Input: part model. Units: mm. Frame: model coordinates. A direction names the side the tool comes from. Coordinates: 2 decimals unless noted, no trailing zeros. Write each loop counter-clockwise with the first axis right and the second up, starting at its lowest first coordinate (ties: lowest second). Pieces come first, ordered by that corner, then holes. Notation, with made-up numbers: M -30.5,59 L 1.5,59 A27 cw 1.5,92 Z; hole C 74,63 d4. An arc over 180 degrees is marked long. Use one line per item in the form item = value.
from build123d import *

# Parameters (mm, degrees)
F0_W     = 30
F0_H     = 154.5
F0_H_2   = 30
F0_W_2   = 190
F0_H_3   = 184.5
F1_DEPTH = 800
F3_DEPTH = 50
F5_DEPTH = 50


with BuildPart() as f1:
    # F0 (on Front) → F1 (new body)
    with BuildSketch(Plane.XZ):
        with Locations((-15, 77.25)):
            Rectangle(F0_W, F0_H)
        with Locations((-15, 169.5)):
            Rectangle(F0_W, F0_H_2)
        with Locations((-125, 169.5)):
            Rectangle(F0_W_2, F0_H_2)
        with Locations((-235, 169.5)):
            Rectangle(F0_W, F0_H_2)
        with Locations((-235, 261.75)):
            Rectangle(F0_W, F0_H)
        with Locations((-235, 354)):
            Rectangle(F0_W, F0_H_2)
        with Locations((-345, 354)):
            Rectangle(F0_W_2, F0_H_2)
        with Locations((-455, 354)):
            Rectangle(F0_W, F0_H_2)
        with Locations((-455, 446.25)):
            Rectangle(F0_W, F0_H)
        with Locations((-455, 538.5)):
            Rectangle(F0_W, F0_H_2)
        with Locations((-565, 538.5)):
            Rectangle(F0_W_2, F0_H_2)
        with Locations((-675, 538.5)):
            Rectangle(F0_W, F0_H_2)
        with Locations((-675, 645.75)):
            Rectangle(F0_W, F0_H_3)
    extrude(amount=F1_DEPTH)

    # F2 (on face) → F3 (join)
    with BuildSketch(Plane.XZ.offset(800)):
        Polygon((-690, 738), (-690, 523.5), (-590, 439.636364), (-590, 700.658275), (-590, 738), align=None)
        Polygon((-590, 439.636364), (-690, 523.5), (-690, 439.636364), align=None)
        Polygon((-590, 700.658275), (-590, 439.636364), (-100, 28.704545), (-100, 289.726456), align=None)
        Polygon((-100, 289.726456), (-100, 28.704545), (-100, -200), (0, -200), (0, 289.726456), align=None)
    extrude(amount=F3_DEPTH)

    # F4 (on face) → F5 (join)
    with BuildSketch(Plane(origin=(0, 0, 0), x_dir=(-1, 0, 0), z_dir=(0, 1, 0))):
        Polygon((0, 289.726456), (0, -200), (100, -200), (100, 28.704545), (100, 289.726456), align=None)
        Polygon((100, 289.726456), (100, 28.704545), (590, 439.636364), (590, 700.658275), align=None)
        Polygon((590, 700.658275), (590, 439.636364), (690, 439.636364), (690, 738), (590, 738), align=None)
    extrude(amount=F5_DEPTH)


solid = f1.part
(1) Section query B-B on x = -635.5. Return the cut outline in (y, z), plus the area to 3 significant figures.
Computed:
outline = M -850,439.64 L -800,439.64 L -800,523.5 L 0,523.5 L 0,439.64 L 50,439.64 L 50,738 L 0,738 L 0,553.5 L -800,553.5 L -800,738 L -850,738 Z
area = 53,800 mm^2
(2) First-contact query: pin 1 Ø8 at (y, z) = (-607.5, 487) entering from +X; pin 2 Ø8 at (y, z) = (-238.5, 349) entering from -X; pin 3 Ø1.5 at (y, z) = (-654, 598.5) entering from +X. Flat tips, straight axial feed; report the tip coordinate or a pass-through.
Computed:
pin_1 = -440
pin_2 = -470
pin_3 = -660
(3) Section query C-C on y = -97. Return the cut outline in (x, z).
Computed:
outline = M -690,523.5 L -470,523.5 L -470,339 L -250,339 L -250,154.5 L -30,154.5 L -30,0 L 0,0 L 0,184.5 L -220,184.5 L -220,369 L -440,369 L -440,553.5 L -660,553.5 L -660,738 L -690,738 Z
(4) Section query D-D on z = 537. Return the cut outline in (x, y).
Computed:
outline = M -690,-850 L -394.85,-850 L -394.85,-800 L -440,-800 L -440,0 L -394.85,0 L -394.85,50 L -690,50 Z
(5) Pull-direction query (Y, two-part tool) for faces 5 (the flat face through (-321, -850, 341)), 6 (the flat face through (-548, -394, 553.5)), 7 (the flat face through (-348.43, 24.65, 498.07)); classes: pulls with the +Y half, pulls with the -Y half, needs draft (parallel to the pull), parting line crosses it, or undercut.
Computed:
face_5 = pulls with the -Y half
face_6 = undercut
face_7 = needs draft
(6) Set-up query: faces 1 (the flat face through (-440, -394, 460)), 2 (the flat face through (-100, -825, -84)), 3 (the flat face through (-590, -825, 719)), 4 (the flat face through (-554, 0, 453)). Return all of +Z, -Z, +X, -X, +Y, -Y with unobstructed straight access to the full face (end or side cutting, diameter ignored); none if empty.
Computed:
face_1 = +Z, +X
face_2 = -Z, -X, +Y, -Y
face_3 = +Z, +X, +Y, -Y
face_4 = -Z, -X
(7) Line query: probe 1 along Y at (x, z) = (-36, -70); probe 2 along Z at (x, y) = (-193, -144); probe 3 along Z at (x, y) = (-468, -617.5). Output: solid intervals per line, ascending.
Computed:
probe_1 = -850 to -800, 0 to 50
probe_2 = 154.5 to 184.5
probe_3 = 339 to 553.5
(8) Section query A-A on z = -73. Return the cut outline in (x, y), plus the area to 3 significant figures.
Computed:
outline = M -100,-850 L 0,-850 L 0,-800 L -100,-800 Z; M -100,0 L 0,0 L 0,50 L -100,50 Z
area = 10,000 mm^2
